Here's how the part is built. I have some questions about the finished solid (model axes, mm). Face numbers are marked on the shaded views. A direction names the side the tool comes from. Round coordinates to 2 decimals unless told otherwise and drop trailing zeros. Order: outer loops, then holes, each group sorted by start corner. A loop starts at its lowest first (then second) coordinate and runs counter-clockwise, first axis right, second up.
```python
from build123d import *

# Parameters (mm, degrees)
SKETCH1_W           = 91.4146
SKETCH1_H           = 199.9996
BOSS_EXTRUDE1_DEPTH = 5.0038
BOSS_EXTRUDE2_DEPTH = 56.3118
FILLET1_R           = 15.0114
CUT_EXTRUDE1_REACH  = 7.004
SKETCH3_R           = 2.1082
FILLET2_R           = 3.81
SKETCH5_R           = 12.7
BOSS_EXTRUDE3_DEPTH = 66.675
FILLET3_R           = 5.08
SKETCH6_R           = 5.588
BOSS_EXTRUDE4_DEPTH = 16.1544


with BuildPart() as part:
    # Sketch1 → Boss-Extrude1 (new body)
    with BuildSketch(Plane(origin=(0, 0, 0), x_dir=(1, 0, 0), z_dir=(0, 1, 0))):
        Rectangle(SKETCH1_W, SKETCH1_H)
    extrude(amount=BOSS_EXTRUDE1_DEPTH)

    # Sketch2 → Boss-Extrude2 (add)
    with BuildSketch(Plane(origin=(0, 5.0038, 0), x_dir=(1, 0, 0), z_dir=(0, 1, 0))):
        with BuildLine():
            Line((-24.1173, 75.7047), (24.1173, 75.7047))
            ThreePointArc((24.1173, 75.7047), (39.383735406, 69.381135406), (45.7073, 54.1147))
            Line((45.7073, 54.1147), (45.7073, -54.1147))
            ThreePointArc((45.7073, -54.1147), (39.383735406, -69.381135406), (24.1173, -75.7047))
            Line((24.1173, -75.7047), (-24.1173, -75.7047))
            ThreePointArc((-24.1173, -75.7047), (-39.383735406, -69.381135406), (-45.7073, -54.1147))
            Line((-45.7073, -54.1147), (-45.7073, 54.1147))
            ThreePointArc((-45.7073, 54.1147), (-39.383735406, 69.381135406), (-24.1173, 75.7047))
        make_face()
    extrude(amount=BOSS_EXTRUDE2_DEPTH)

    # Fillet1
    fillet1_edges = [part.edges().sort_by_distance(p)[0] for p in [
        (-39.383735406, 61.3156, -69.381135406),
        (-45.7073, 61.3156, 0),
        (-39.383735406, 61.3156, 69.381135406),
        (0, 61.3156, 75.7047),
        (39.383735406, 61.3156, 69.381135406),
        (45.7073, 61.3156, 0),
        (39.383735406, 61.3156, -69.381135406),
        (0, 61.3156, -75.7047),
    ]]
    fillet(fillet1_edges, radius=FILLET1_R)

    # Sketch3 → Cut-Extrude1 (cut, up to next)
    with BuildSketch(Plane(origin=(0, 5.0038, 0), x_dir=(1, 0, 0), z_dir=(0, 1, 0)), mode=Mode.PRIVATE) as cut_extrude1_sk1:
        with Locations((25.9969, 94.996)):
            Circle(SKETCH3_R)
    cut_extrude1_tool1 = extrude(cut_extrude1_sk1.sketch, amount=-CUT_EXTRUDE1_REACH, mode=Mode.PRIVATE) & part.part
    add(cut_extrude1_tool1.solids().sort_by_distance((25.9969, 5.0038, -94.996))[0], mode=Mode.SUBTRACT)
    # Sketch3 → Cut-Extrude1 (cut, up to next)
    with BuildSketch(Plane(origin=(0, 5.0038, 0), x_dir=(1, 0, 0), z_dir=(0, 1, 0)), mode=Mode.PRIVATE) as cut_extrude1_sk2:
        with Locations((-25.9969, 94.996)):
            Circle(SKETCH3_R)
    cut_extrude1_tool2 = extrude(cut_extrude1_sk2.sketch, amount=-CUT_EXTRUDE1_REACH, mode=Mode.PRIVATE) & part.part
    add(cut_extrude1_tool2.solids().sort_by_distance((-25.9969, 5.0038, -94.996))[0], mode=Mode.SUBTRACT)
    # Sketch3 → Cut-Extrude1 (cut, up to next)
    with BuildSketch(Plane(origin=(0, 5.0038, 0), x_dir=(1, 0, 0), z_dir=(0, 1, 0)), mode=Mode.PRIVATE) as cut_extrude1_sk3:
        with Locations((25.9969, -94.996)):
            Circle(SKETCH3_R)
    cut_extrude1_tool3 = extrude(cut_extrude1_sk3.sketch, amount=-CUT_EXTRUDE1_REACH, mode=Mode.PRIVATE) & part.part
    add(cut_extrude1_tool3.solids().sort_by_distance((25.9969, 5.0038, 94.996))[0], mode=Mode.SUBTRACT)
    # Sketch3 → Cut-Extrude1 (cut, up to next)
    with BuildSketch(Plane(origin=(0, 5.0038, 0), x_dir=(1, 0, 0), z_dir=(0, 1, 0)), mode=Mode.PRIVATE) as cut_extrude1_sk4:
        with Locations((-25.9969, -94.996)):
            Circle(SKETCH3_R)
    cut_extrude1_tool4 = extrude(cut_extrude1_sk4.sketch, amount=-CUT_EXTRUDE1_REACH, mode=Mode.PRIVATE) & part.part
    add(cut_extrude1_tool4.solids().sort_by_distance((-25.9969, 5.0038, 94.996))[0], mode=Mode.SUBTRACT)

    # Fillet2
    fillet2_edges = [part.edges().sort_by_distance(p)[0] for p in [
        (45.7073, 2.5019, 99.9998),
        (-45.7073, 2.5019, 99.9998),
        (-45.7073, 2.5019, -99.9998),
        (45.7073, 2.5019, -99.9998),
    ]]
    fillet(fillet2_edges, radius=FILLET2_R)

    # Sketch5 → Boss-Extrude3 (add)
    with BuildSketch(Plane.XY.offset(75.7047)):
        with Locations((0, 27.8638)):
            Circle(SKETCH5_R)
    extrude(amount=BOSS_EXTRUDE3_DEPTH)

    # Fillet3
    fillet3_edges = [part.edges().sort_by_distance(p)[0] for p in [
        (-12.7, 27.8638, 142.3797),
    ]]
    fillet(fillet3_edges, radius=FILLET3_R)

    # Sketch6 → Boss-Extrude4 (add)
    with BuildSketch(Plane(origin=(0, 0, -75.7047), x_dir=(-1, 0, 0), z_dir=(0, 0, -1))):
        with Locations((0, 32.269838727)):
            Circle(SKETCH6_R)
    extrude(amount=BOSS_EXTRUDE4_DEPTH)


solid = part.part
```
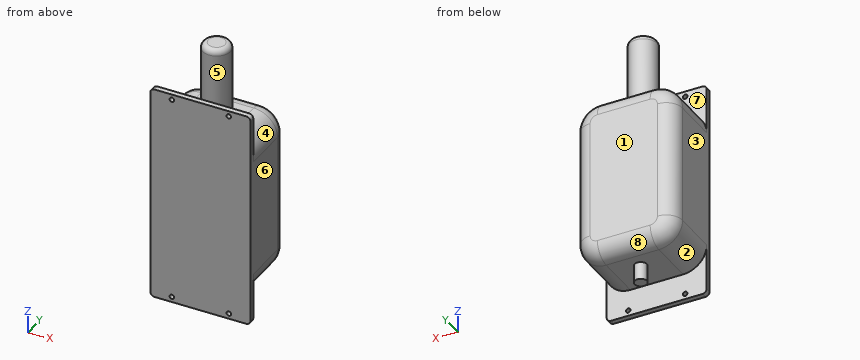
1. If we section it at D-D, the plane z = 106: Write out the boundary of the cut face in (x, y).
Evaluation:
outline: circle Ø25.4 at (0, 27.86)
2. If we section it at C-C, the plane x = 0: Write out the boundary of the cut face in (y, z).
Evaluation:
outline: (0, -100) - (5, -100) - (5, -75.7) - (26.68, -75.7) - (26.68, -91.86) - (37.86, -91.86) - (37.86, -75.7) - (46.3, -75.7) arc R15.01 ccw to (61.32, -60.69) - (61.32, 60.69) arc R15.01 ccw to (46.3, 75.7) - (40.56, 75.7) - (40.56, 137.3) arc R5.08 ccw to (35.48, 142.38) - (20.24, 142.38) arc R5.08 ccw to (15.16, 137.3) - (15.16, 75.7) - (5, 75.7) - (5, 100) - (0, 100) - close
3. If we section it at B-B, the plane z = 31: Write out the boundary of the cut face in (x, y).
Evaluation:
outline: (-45.71, 0) - (45.71, 0) - (45.71, 46.3) arc R15.01 ccw to (30.7, 61.32) - (-30.7, 61.32) arc R15.01 ccw to (-45.71, 46.3) - close
4. I need wall thicknesses on probe 1 along Z at (x, y) = (-24, 35); probe 2 along Y at (x, z) = (-30.5, 85.5); probe 3 along Z at (x, y) = (3, 30). Which ranges of each line are inside material? Lowest first, please.
Evaluation:
probe 1: z = -75.7 to 75.7
probe 2: y = 0 to 5
probe 3: z = -91.86 to 142.38
5. I'm going to push flat-ended pins straight in: P1, Ø5.5, axis at x = 1.5, y = 34.5, coming from the -Z side; P2, Ø10, axis at x = -25, z = 13.5, coming from the -Y side; P3, Ø10, axis at x = 34, y = 11.5, coming from the -Z side; P4, Ø14, axis at x = -11, z = 79, coming from the +Y side. Where does each tip first touch, or does it pass through?
Evaluation:
P1: stops at z = -91.86
P2: stops at y = 0
P3: stops at z = -75.15
P4: stops at y = 56.18
6. On a 3-axis mill with a long thin cutter (end or side, diameter ignored), from which of +Z, -Z, +X, -X, +Y, -Y can I reach the whole of each face in a straight line? I mean the marked faces 1, 2, 3, 4 and 5. Say none if no direction works.
Evaluation:
face 1: +Z, -Z, +X, -X, +Y
face 2: -Z, -X, +Y
face 3: +Z, -Z, -X, +Y, -Y
face 4: +Z, +X, +Y
face 5: +Z
7. If we mould it in two halves opening along Y, with no side actions, what happens to the marked faces 6, 7 and 8? For each: released by +Y, released by -Y, zero draft, split by the parting line, or undercut.
Evaluation:
face 6: zero draft
face 7: undercut
face 8: released by +Y
8. If we section it at A-A, the plane x = 18.5: Write out the boundary of the cut face in (y, z), and give its area (3 significant figures).
Evaluation:
outline: (0, -100) - (5, -100) - (5, -75.7) - (46.3, -75.7) arc R15.01 ccw to (61.32, -60.69) - (61.32, 60.69) arc R15.01 ccw to (46.3, 75.7) - (5, 75.7) - (5, 100) - (0, 100) - close
area: 9,430 mm2
